The listing builds one solid part. Answer for the finished solid, in the listing's coordinates (mm). A direction names the side the tool comes from. Round coordinates to 2 decimals unless told otherwise and drop trailing zeros. Write each loop counter-clockwise with the first axis right and the second up, starting at its lowest first coordinate (ties: lowest second). Pieces come first, ordered by that corner, then holes. Notation, with made-up numbers: (-19.75, 83.5) - (-13.75, 83.5) arc R21 cw to (-13.75, 102.5) - close; hole circle Ø4 at (-22, 87). An arc over 180 degrees is marked (long way). Answer in a Markdown table with one row per item.
from build123d import *

# Parameters (mm, degrees)
BOSS_EXTRUDE1_DEPTH = 160
BOSS_EXTRUDE2_DEPTH = 110


with BuildPart() as part:
    # Sketch1 → Boss-Extrude1 (new body)
    with BuildSketch(Plane.XY):
        with BuildLine():
            ThreePointArc((-19.364916731, 5), (-19.840593925, 2.52008585), (-20, 0))
            Line((-20, 0), (20, 0))
            ThreePointArc((20, 0), (2.52008585, 19.840593925), (-19.364916731, 5))
        make_face()
        with BuildLine():
            Line((20, 0), (-20, 0))
            ThreePointArc((-20, 0), (-19.840593925, -2.52008585), (-19.364916731, -5))
            ThreePointArc((-19.364916731, -5), (2.52008585, -19.840593925), (20, 0))
        make_face()
    extrude(amount=BOSS_EXTRUDE1_DEPTH)

    # Sketch1_3 → Boss-Extrude2 (add)
    with BuildSketch(Plane.XY):
        with BuildLine():
            Line((-24.364916731, 5), (-24.364916731, 0))
            Line((-24.364916731, 0), (-20, 0))
            ThreePointArc((-20, 0), (-19.840593925, 2.52008585), (-19.364916731, 5))
            Line((-19.364916731, 5), (-24.364916731, 5))
        make_face()
        with BuildLine():
            Line((-20, 0), (-24.364916731, 0))
            Line((-24.364916731, 0), (-24.364916731, -5))
            Line((-24.364916731, -5), (-19.364916731, -5))
            ThreePointArc((-19.364916731, -5), (-19.840593925, -2.52008585), (-20, 0))
        make_face()
    extrude(amount=BOSS_EXTRUDE2_DEPTH)


solid = part.part
(1) Section B-B (z = 35.5) is taken. Give the vertices of the cut face in (x, y).
Checked values:
| item | result |
|---|---|
| outline | (-24.36, -5) - (-19.36, -5) arc R20 ccw (long way) to (-19.36, 5) - (-24.36, 5) - close |
(2) Flat-ended cylindrical pins translate along their axes: pin 1 (2.5 mm diameter, centred on x = -22.5, z = 79, fed in from -Y); pin 2 (1.5 mm diameter, centred on x = -22, y = 0.5, fed in from +Z); pin 3 (6 mm diameter, centred on x = 12.5, z = 128, fed in from -Y). Find the tip coordinate at first contact, or state that the pin passes through.
Checked values:
| item | result |
|---|---|
| pin 1 | stops at y = -5 |
| pin 2 | stops at z = 110 |
| pin 3 | stops at y = -17.6 |
(3) Section A-A (y = 12) is taken. Give the vertices of the cut face in (x, z).
Checked values:
| item | result |
|---|---|
| outline | (-16, 0) - (16, 0) - (16, 160) - (-16, 160) - close |
(4) Find the intervals of material crossed by line 1 (Y direction, x = -19.5, z = 101); line 2 (X direction, y = 1, z = 82); line 3 (Y direction, x = 16, z = 81), in increasing order.
Checked values:
| item | result |
|---|---|
| line 1 | y = -5 to 5 |
| line 2 | x = -24.36 to 19.97 |
| line 3 | y = -12 to 12 |
(5) For faces 1 (the flat face through (-22, 5, 54)), 2 (the flat face through (-22, -5, 54)), 3 (the flat face through (-24.365, 0, 54)), determine the directions among +Z, -Z, +X, -X, +Y, -Y from which every point of the face is accessible in a straight line to the end or side of a thin tool.
Checked values:
| item | result |
|---|---|
| face 1 | +Z, -Z, -X, +Y |
| face 2 | +Z, -Z, -X, -Y |
| face 3 | +Z, -Z, -X, +Y, -Y |
